from build123d import *

# Parameters (mm, degrees)
F0_W     = 100
F0_H     = 35
F1_DEPTH = 18
F3_D     = 12
F4_R     = 12.7
F5_DEPTH = 19
F6_R     = 25
F6_R_2   = 12.7
F7_DEPTH = 5.5
F8_R     = 2.5
F9_DEPTH = 3


with BuildPart() as f1:
    # F0 (on Top) → F1 (new body)
    with BuildSketch(Plane.XY):
        Rectangle(F0_W, F0_H)
    extrude(amount=-F1_DEPTH)

    # F3 (through all)
    with Locations(Plane.XY):
        with Locations((-35, 0), (35, 0)):
            Hole(F3_D / 2)

    # F4 (on face) → F5 (join)
    with BuildSketch(Plane.XY):
        Circle(F4_R)
    extrude(amount=F5_DEPTH)

    # F6 (on face) → F7 (join)
    with BuildSketch(Plane.XY.offset(19)):
        Circle(F6_R)
        Circle(F6_R_2, mode=Mode.SUBTRACT)
        Circle(F6_R_2)
    extrude(amount=F7_DEPTH)

    # F8 (on face) → F9 (join)
    with BuildSketch(Plane.XY.offset(24.5)):
        Circle(F8_R)
    extrude(amount=F9_DEPTH)


solid = f1.part
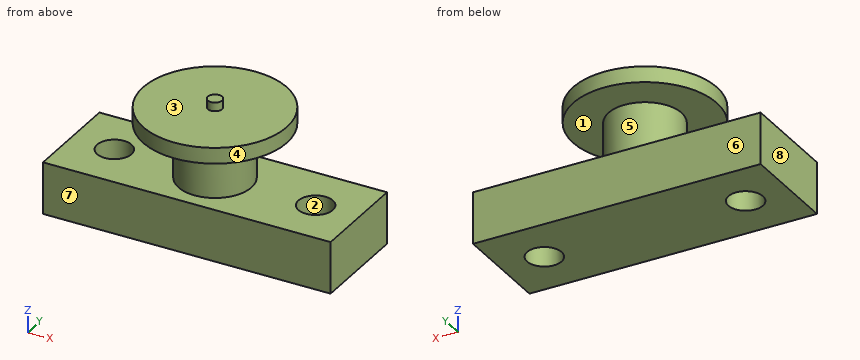
For this review, take the finished solid that the model builds, in its own axes (mm). Face numbers are marked on the shaded views. A direction names the side the tool comes from. Round coordinates to 2 decimals unless told otherwise and drop trailing zeros. Loops run counter-clockwise (first coordinate to the right, second up) from the corner with the lowest first, then second, coordinate; pieces in that order, holes last. Notation, with made-up numbers: (-6, 47.25) - (37, 47.25) arc R20 ccw to (37, 78.25) - close; hole circle Ø5 at (-2.75, -23.5). An arc over 180 degrees is marked (long way). One line per question, with ' | ' between items.
Q1. Take a section at D-D (z = -7.5). Give the boundary of the cut face in (x, y), and give its area (3 significant figures).
Taken from the geometry:
outline: (-50, -17.5) - (50, -17.5) - (50, 17.5) - (-50, 17.5) - close; hole circle Ø12 at (-35, 0); hole circle Ø12 at (35, 0) | area: 3,270 mm²
Q2. Take a section at B-B (y = -14). Give the boundary of the cut face in (x, z), and give its area (3 significant figures).
Taken from the geometry:
outline: (-50, -18) - (50, -18) - (50, 0) - (-50, 0) - close; (-20.71, 19) - (20.71, 19) - (20.71, 24.5) - (-20.71, 24.5) - close | area: 2,030 mm²
Q3. For line 1 along Y through (x, z) = (35, -7.5); line 2 along Z through (x, y) = (12.5, -10); line 3 along Z through (x, y) = (2, -19.5), list the stretches that pass through material, from the lowest coordinate up. Write a range as [from, to].
Taken from the geometry:
line 1: y = [-17.5, -6], [6, 17.5] | line 2: z = [-18, 0], [19, 24.5] | line 3: z = [19, 24.5]
Q4. Tool access review of the marked faces 4, 5, 6, 7 and 8: name each direction out of +Z, -Z, +X, -X, +Y, -Y from which nothing blocks a thin tool from reaching the whole face with its end or side.
Taken from the geometry:
face 4: +Z | face 5: none | face 6: -Z, +X, -X, +Y | face 7: -Z, +X, -X, -Y | face 8: +Z, -Z, -X, +Y, -Y
Q5. Take a section at C-C (y = 0). Give the boundary of the cut face in (x, z), and give its area (3 significant figures).
Taken from the geometry:
outline: (-50, -18) - (-41, -18) - (-41, 0) - (-50, 0) - close; (-29, -18) - (29, -18) - (29, 0) - (12.7, 0) - (12.7, 19) - (25, 19) - (25, 24.5) - (2.5, 24.5) - (2.5, 27.5) - (-2.5, 27.5) - (-2.5, 24.5) - (-25, 24.5) - (-25, 19) - (-12.7, 19) - (-12.7, 0) - (-29, 0) - close; (41, -18) - (50, -18) - (50, 0) - (41, 0) - close | area: 2,140 mm²
Q6. The part is to be moulded in two halves that separate along Z. For the marked faces 1, 2 and 3, say which applies: released by +Z, released by -Z, zero draft, split by the parting line, or undercut.
Taken from the geometry:
face 1: undercut | face 2: zero draft | face 3: released by +Z
Q7. For pin 1 (12 mm diameter, centred on y = -5, z = 4.5, fed in from -X); pin 2 (10.5 mm diameter, centred on x = -8.5, y = 7, fed in from +Z); pin 3 (15.5 mm diameter, centred on x = -35, y = 0, fed in from +Z); pin 4 (4 mm diameter, centred on y = -1.5, z = 12.5, fed in from +X), all flat-tipped, find the tip position at first contact; note any pin that passes through.
Taken from the geometry:
pin 1: stops at x = -50 | pin 2: stops at z = 24.5 | pin 3: stops at z = 0 | pin 4: stops at x = 12.7
Q8. Take a section at A-A (x = 35). Give the boundary of the cut face in (y, z), and give its area (3 significant figures).
Taken from the geometry:
outline: (-17.5, -18) - (-6, -18) - (-6, 0) - (-17.5, 0) - close; (6, -18) - (17.5, -18) - (17.5, 0) - (6, 0) - close | area: 414 mm²
